from build123d import *

# Parameters (mm, degrees)
SKETCH1_R           = 12.78
SKETCH1_R_2         = 2.78
BOSS_EXTRUDE1_DEPTH = 2.5


with BuildPart() as part:
    # Sketch1 → Boss-Extrude1 (new body, symmetric)
    with BuildSketch(Plane.XY):
        with BuildLine():
            ThreePointArc((12.78, 150), (0, 137.22), (-12.78, 150))
            Line((-12.78, 150), (-12.78, 0))
            ThreePointArc((-12.78, 0), (0, 12.78), (12.78, 0))
            Line((12.78, 0), (12.78, 150))
        make_face()
        with Locations((0, 150)):
            Circle(SKETCH1_R)
        with Locations((0, 150)):
            Circle(SKETCH1_R_2, mode=Mode.SUBTRACT)
        Circle(SKETCH1_R)
        Circle(SKETCH1_R_2, mode=Mode.SUBTRACT)
    extrude(amount=BOSS_EXTRUDE1_DEPTH, both=True)


solid = part.part
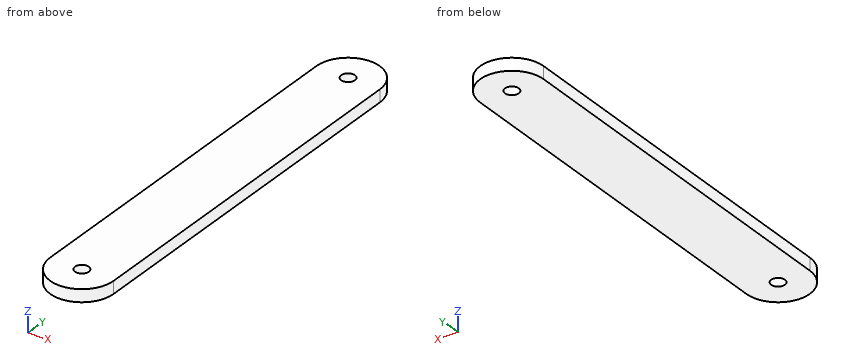
Can you work these out from the model? Positions are in its coordinate system, mm. Round coordinates to 2 decimals unless told otherwise and drop trailing zeros. Write each loop counter-clockwise with the first axis right and the second up, starting at its lowest first coordinate (ties: lowest second). Pieces come first, ordered by that corner, then holes. Notation, with made-up numbers: (18.5, -8) -> (54.5, -8) arc R24 ccw to (54.5, 8) -> close; hole circle Ø10 at (-10.75, -32.75). An arc over 180 degrees is marked (long way). One line per question, with ' | ' between items. Start each with the question number.
1) Suppose I cut it at B-B on z = 1.7. Write out the boundary of the cut face in (x, y), then the cut area to 3 significant figures.
2) I need wall thicknesses on line 1 (Y direction, x = 0, z = 0.5); line 2 (X direction, y = 150, z = -0.65); line 3 (Y direction, x = -2.25, z = 1.3). Which ranges of each line are inside material? Lowest first, please. Write a range as [from, to].
3) Suppose I cut it at C-C on x = 9.5. Write out the boundary of the cut face in (y, z), then the cut area to 3 significant figures.
4) Suppose I cut it at A-A on x = 0. Write out the boundary of the cut face in (y, z).
Return value:
1) outline: (-12.78, 0) arc R12.78 ccw to (12.78, 0) -> (12.78, 150) arc R12.78 ccw to (-12.78, 150) -> close; hole circle Ø5.56 at (0, 0); hole circle Ø5.56 at (0, 150) | area: 4,300 mm2
2) line 1: y = [-12.78, -2.78], [2.78, 147.22], [152.78, 162.78] | line 2: x = [-12.78, -2.78], [2.78, 12.78] | line 3: y = [-12.58, -1.63], [1.63, 148.37], [151.63, 162.58]
3) outline: (-8.55, -2.5) -> (158.55, -2.5) -> (158.55, 2.5) -> (-8.55, 2.5) -> close | area: 835 mm2
4) outline: (-12.78, -2.5) -> (-2.78, -2.5) -> (-2.78, 2.5) -> (-12.78, 2.5) -> close; (2.78, -2.5) -> (147.22, -2.5) -> (147.22, 2.5) -> (2.78, 2.5) -> close; (152.78, -2.5) -> (162.78, -2.5) -> (162.78, 2.5) -> (152.78, 2.5) -> close
